Can you work these out from the drawing? Everything is in mm from the part's minimum corner. Coordinates: 2 decimals unless noted, no trailing zeros. Order: outer loops, then holes, each group sorted by start corner. A loop starts at its lowest first (then second) coordinate and runs counter-clockwise, first axis right, second up. Notation, with made-up numbers: (21, -12.75) -> (34, -12.75) arc R23 cw to (34, 26.25) -> close; hole circle Ø5 at (-9, 64.25). An arc over 180 degrees is marked (long way). Return JSON: item names as keys, results as strings. Group by question number.
1) If I drill on probe 1 along X at (y, z) = (5.25, 84), over which ranges is the centre line in solid material (lowest first)? Write a range as from..to.
2) If we section it at A-A, the plane y = 5.25: State how many separate pieces and enclosed holes the cut face has, then the cut area to 3 significant figures.
3) If we section it at B-B, the plane z = 69.5: Please give me the cut outline in (x, y), then the cut area to 3 significant figures.
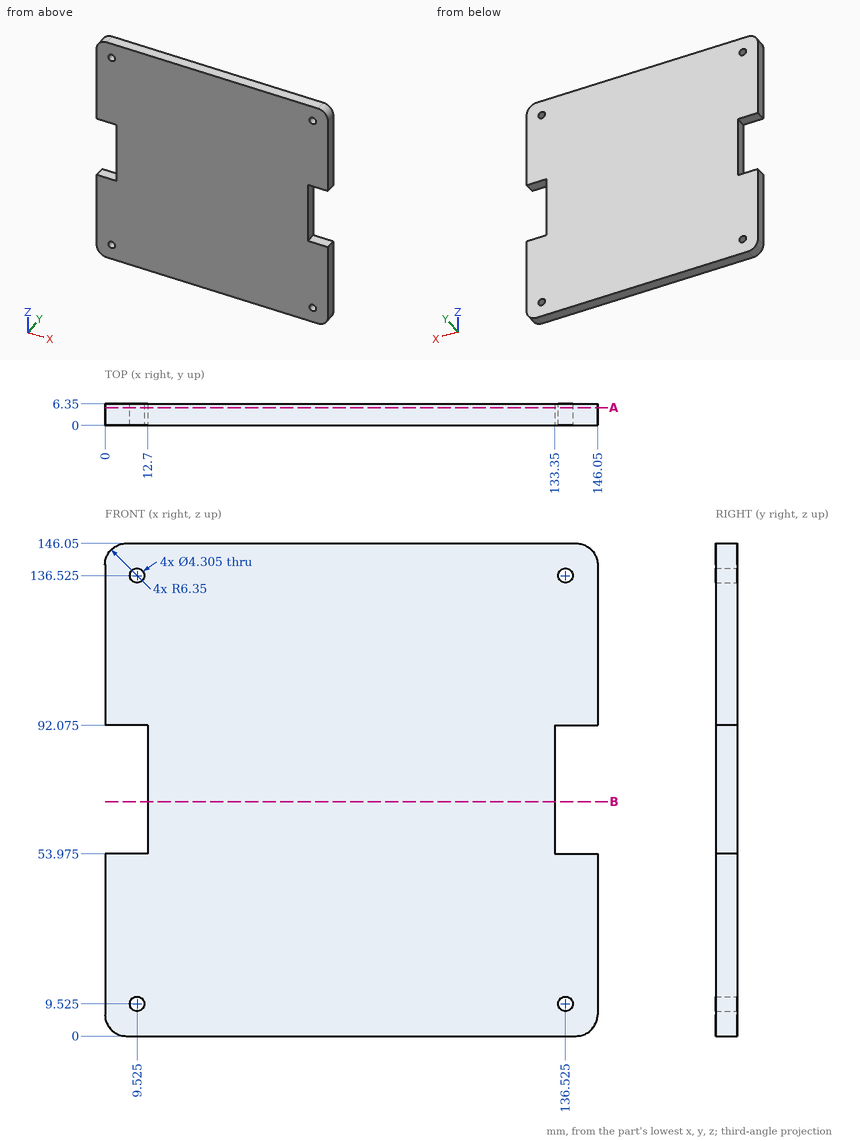
Result sheet:
{
 "1": {"probe 1": "x = 12.7..133.35"},
 "2": {"separate pieces": "1", "enclosed holes": "4", "area": "20,300 mm2"},
 "3": {"outline": "(12.7, 0) -> (133.35, 0) -> (133.35, 6.35) -> (12.7, 6.35) -> close", "area": "766 mm2"}
}
